```python
from build123d import *

# Parameters (mm, degrees)
SKETCH1_W                          = 140.716
SKETCH1_H                          = 55.88
BOSS_EXTRUDE1_DEPTH                = 3.175
SKETCH2_W                          = 3.2258
SKETCH2_H                          = 6.35
HOLES_FOR_TABS_DEPTH               = 4.175
SKETCH3_W                          = 3.2258
SKETCH3_H                          = 6.35
CUT_FOR_TABS_NOSEPANEL_DEPTH       = 4.175
SKETCH5_R                          = 0.508
CUT_FOR_OPTIONAL_MOTORS_EARS_DEPTH = 4.175
BOSS_EXTRUDE2_DEPTH                = 3.175
SKETCH7_R                          = 1.7145
CUT_FOR_ARDUINO_MOUNT_HOLES_DEPTH  = 4.175


with BuildPart() as part:
    # Sketch1 → Boss-Extrude1 (new body)
    with BuildSketch(Plane.XY):
        Rectangle(SKETCH1_W, SKETCH1_H)
    extrude(amount=BOSS_EXTRUDE1_DEPTH)

    # Sketch2 → holes for tabs (cut, through all)
    with BuildSketch(Plane.XY.offset(3.175)):
        with Locations((-65.5701, 18.415)):
            Rectangle(SKETCH2_W, SKETCH2_H)
        with Locations((-65.5701, -19.685)):
            Rectangle(SKETCH2_W, SKETCH2_H)
    holes_for_tabs = extrude(amount=-HOLES_FOR_TABS_DEPTH, mode=Mode.SUBTRACT)

    # Mirror1: holes for tabs across plane
    add(holes_for_tabs.mirror(Plane(origin=(0, 0, 0), x_dir=(0, 0, 1), z_dir=(1, 0, 0))), mode=Mode.SUBTRACT)

    # Sketch3 → cut for tabs, nosepanel (cut, through all)
    with BuildSketch(Plane.XY.offset(3.175)):
        with Locations((0, 18.415547881)):
            Rectangle(SKETCH3_W, SKETCH3_H)
        with Locations((0, -13.264075424)):
            Rectangle(SKETCH3_W, SKETCH3_H)
    extrude(amount=-CUT_FOR_TABS_NOSEPANEL_DEPTH, mode=Mode.SUBTRACT)

    # Sketch5 → cut for optional motors (ears) (cut, through all)
    with BuildSketch(Plane.XY.offset(3.175)):
        with Locations((-50.8, -18.796)):
            Circle(SKETCH5_R)
        with Locations((-50.8, 9.144)):
            Circle(SKETCH5_R)
        Polygon((-44.45, 6.604), (-57.15, 6.604), (-57.15, -16.256), (-53.975, -16.256), (-53.975, -17.653), (-47.625, -17.653), (-47.625, -16.256), (-44.45, -16.256), align=None)
    cut_for_optional_motors_ears = extrude(amount=-CUT_FOR_OPTIONAL_MOTORS_EARS_DEPTH, mode=Mode.SUBTRACT)

    # Mirror2: cut for optional motors (ears) across plane
    add(cut_for_optional_motors_ears.mirror(Plane(origin=(0, 0, 0), x_dir=(0, 0, 1), z_dir=(1, 0, 0))), mode=Mode.SUBTRACT)

    # Sketch6 → Boss-Extrude2 (add)
    with BuildSketch(Plane.XY.offset(3.175)):
        Polygon((0, -27.94), (0, -36.218644949), (-23.051937452, -36.218644949), (-37.953832941, -27.94), align=None)
        Polygon((0, 27.94), (0, 43.18), (-25.4, 43.18), (-50.8, 27.94), align=None)
    boss_extrude2 = extrude(amount=-BOSS_EXTRUDE2_DEPTH)

    # Mirror3: Boss-Extrude2 across plane
    add(boss_extrude2.mirror(Plane(origin=(0, 0, 0), x_dir=(0, 0, 1), z_dir=(1, 0, 0))))

    # Sketch7 → cut for arduino mount holes (cut, through all)
    with BuildSketch(Plane(origin=(0, 0, 0), x_dir=(-1, 0, 0), z_dir=(0, 0, -1))):
        with Locations((19.154550283, 38.4302)):
            Circle(SKETCH7_R)
        with Locations((-9.293449717, 38.4302)):
            Circle(SKETCH7_R)
        with Locations((24.234550283, -13.97)):
            Circle(SKETCH7_R)
        with Locations((-24.279449717, -12.319)):
            Circle(SKETCH7_R)
    extrude(amount=-CUT_FOR_ARDUINO_MOUNT_HOLES_DEPTH, mode=Mode.SUBTRACT)


solid = part.part
```
Build history of the part. All positions in model axes, mm. A direction names the side the tool comes from. Give positions to 0.01 mm unless a question says otherwise; leave off trailing zeros. Order: outer loops, then holes, each group sorted by start corner. A loop starts at its lowest first (then second) coordinate and runs counter-clockwise, first axis right, second up. Notation, with made-up numbers: M -32,-38 L -6,-38 A21 ccw -6,-24 Z; hole C -25,61 d5. An arc over 180 degrees is marked long. Return JSON: item names as keys, results as strings.
Q1. 3-axis set-ups, long thin cutter, end or side, ignore diameter. For faces 1 (the face through (70.358, 0, 2)), 2 (the face through (60, 27.94, 2)), 3 (the face through (-66, 21.59, 2)): which of +Z, -Z, +X, -X, +Y, -Y reach the whole face in a straight line?
Answer list:
{"face 1": "+Z, -Z, +X, +Y, -Y", "face 2": "+Z, -Z, +X, +Y", "face 3": "+Z, -Z"}
Q2. Wall check: probe 1 along X at (y, z) = (-22.5, 2.6); probe 2 along Y at (x, z) = (-1.5, 2.45); probe 3 along X at (y, z) = (-5.5, 0.8). Give the ranges that are in metal, low to high. Write a range as from..to.
Answer list:
{"probe 1": "x = -70.36..-67.18, -63.96..63.96, 67.18..70.36", "probe 2": "y = -36.22..-16.44, -10.09..15.24, 21.59..43.18", "probe 3": "x = -70.36..-57.15, -44.45..44.45, 57.15..70.36"}
Q3. Flat gauge pins, fed straight in: pin 1 (1.6 mm diameter, centred on x = -56.5, z = 1.5, fed in from -Y); pin 2 (1.6 mm diameter, centred on x = -55.5, z = 1.5, fed in from +Y). Where does each tip first touch, or does it go through?
Answer list:
{"pin 1": "stops at y = -27.94", "pin 2": "stops at y = 27.94"}
Q4. Band-saw the part on D-D (x = -28). Give the cut face in (y, z) (3 decimals), then the cut area to 3 significant figures.
Answer list:
{"outline": "M -33.47,0 L 41.62,0 L 41.62,3.175 L -33.47,3.175 Z", "area": "238 mm^2"}
Q5. Two-plate mould, pull along Y, no slides. Class faces 4 (the face through (-30.399, -32.137, 1.61)), 5 (the face through (-1, 4, 3.175)), 6 (the face through (-17.9, 39.6, 1.6)): pulls with the +Y half, pulls with the -Y half, needs draft (parallel to the pull), parting line crosses it, or undercut.
Answer list:
{"face 4": "pulls with the -Y half", "face 5": "needs draft", "face 6": "undercut"}
Q6. Band-saw the part on B-B (x = 61). Give the cut face in (y, z) (3 decimals).
Answer list:
{"outline": "M -27.94,0 L 27.94,0 L 27.94,3.175 L -27.94,3.175 Z"}
Q7. Band-saw the part on C-C (z = 0.8). Count the separate pieces of the cut face and the enclosed holes in it, then the cut area to 3 significant figures.
Answer list:
{"separate pieces": "1", "enclosed holes": "16", "area": "8,770 mm^2"}
Q8. Band-saw the part on A-A (y = -2). Give the cut face in (x, z) (3 decimals).
Answer list:
{"outline": "M -70.358,0 L -57.15,0 L -57.15,3.175 L -70.358,3.175 Z; M -44.45,0 L 44.45,0 L 44.45,3.175 L -44.45,3.175 Z; M 57.15,0 L 70.358,0 L 70.358,3.175 L 57.15,3.175 Z"}
